Autodesk Inventor part; units mm, degrees
ref_plane "Work Plane1" through (29, 0, 0) normal (0, -1, 0) x (1, 0, 0)
ref_plane "YZ Plane" through (0, 0, 0) normal (1, 0, 0) x (0, 1, 0)
ref_plane "XZ Plane" through (0, 0, 0) normal (0, 1, 0) x (-1, 0, 0)
sketch "Sketch1" plane through (0, 0, 0) normal (0, 0, 1) x (1, 0, 0)
  line L0 (-0.19, 0) -> (20, 0)
  line L1 (20, 0) -> (20, 2.5)
  line L2 (20, 2.5) -> (2.4, 2.5)
  line L3 (2.4, 2.5) -> (1.9091, 2.5)
  line L4 (1.9091, 2.5) -> (0, 2.5)
  line L5 (0, 2.5) -> (0, 4.75)
  line L6 (0, 4.75) -> (-2.75, 4.75)
  line L7 (-2.75, 4.75) -> (-2.75, 1.7321)
  line L8 (-2.75, 1.7321) -> (-1.19, 1.7321)
  line L9 (-1.19, 1.7321) -> (-0.19, 0)
  line L10 (-7.3, 0) -> (24.55, 0)
  line L11 (0, -0.95) -> (0, 5.7)
  line L12 (2.4, 2.5) -> (0, 2.5) construction
  dimension "d1" = 17.6
  dimension "d2" = 0.4909
  dimension "d3" = 2.75
  dimension "d4" = 1.56
  dimension "d5" = 60
  dimension "d6" = 5
  dimension "d7" = 5
  dimension "d8" = 3.4641
  dimension "d9" = 9.5
  dimension "d26" = 20
revolve "Body" add sketch "Sketch1" angle 360 about axis through (-0.19, 0, 0) along (1, 0, 0)
sketch "Sketch2" plane through (-2.75, 0, 0) normal (-1, 0, 0) x (0, 0, 1)
  circle A0 centre (0, 0) radius 1.7321
  line L0 (0, -6.65) -> (0, 6.65)
  line L1 (-6.65, 0) -> (6.65, 0)
  line L2 (1.7321, 0) -> (0.866, -1.5)
  line L3 (0.866, -1.5) -> (-0.866, -1.5)
  line L4 (-0.866, -1.5) -> (-1.7321, 0)
  line L5 (-1.7321, 0) -> (-0.866, 1.5)
  line L6 (-0.866, 1.5) -> (0.866, 1.5)
  line L7 (0.866, 1.5) -> (1.7321, 0)
extrude "Slot" add sketch "Sketch2" against normal up to next contours L7 A0 | A0 L2 | L6 L0 A0 | A0 L0 L3 | L0 L6 A0 | A0 L3 L0 | L4 A0 | A0 L5
fillet "Fillet1" radius 2.37 1 edges at (-2.75, -4.75, 0)
thread "Thread"
chamfer "Chamfer1" distance 0.4908 distance2 0.4908 1 edges at (20, -2.5, 0) measured on face at (20, -0.7379, -0.3873)
ref_plane "Work Plane1" through (29, 0, 0) normal (0, -1, 0) x (1, 0, 0)
fillet "Fillet2" radius 0.45 1 edges at (0, -2.5, 0)
equation "\"d1\" = GEL"
equation "\"d3\" = KOH"
equation "\"d4\" = INTI"
equation "\"d6\" = GD"
equation "\"d7\" = BDM"
equation "\"d8\" = 1.1547 * SW"
equation "\"d9\" = KOD"
equation "\"d26\" = NLG"
equation "\"d30\" = R"
equation "\"d17\" = RR"
equation "\"d13\" = GEL"
equation "\"d15\" = -0.5 * SPD + 0.5 * GD"
equation "\"d16\" = GUL"
equation "\"GD\" = NND"
equation "\"NLG\" = 20"
equation "\"GEL\" = 17.6"
equation "\"KOD\" = 9.5"
equation "\"KOH\" = 2.75"
equation "\"INTI\" = 1.56"
equation "\"GAL\" = 0.61345 * PTC"
equation "\"GUL\" = 0.61345 * PTC"
equation "\"BDM\" = NND"
equation "\"SW\" = 3"
equation "\"RR\" = 2.37"
equation "\"SPD\" = NND - 1.2269 * PTC"
equation "\"R\" = 0.45"
equation "\"TOA\" = 30deg"
equation "\"GD1\" = THREADDIA - 1.2269 * PTC"
equation "\"THREADDIA\" = 5"
equation "\"PTC\" = 0.8"
equation "\"NND\" = 5"
equation "\"KOH1\" = 0.38"
equation "\"E0\" = 3.443"
properties part number "ISO 7380-1 - M5 x 20" material "Steel"
The model under review builds one solid part; all positions refer to its coordinate system, in mm. A direction names the side the tool comes from. Round coordinates to 2 decimals unless told otherwise and drop trailing zeros. Loops run counter-clockwise (first coordinate to the right, second up) from the corner with the lowest first, then second, coordinate; pieces in that order, holes last.
1) Wall thickness on line 1 along Y through (x, z) = (13.5, -0.75); line 2 along Z through (x, y) = (6.5, 0.5); line 3 along X through (y, z) = (2.5, 2.5): over which ranges is each line inside the solid? List them lowest first.
Values follow:
line 1: y = -2.38 to 2.38
line 2: z = -2.45 to 2.45
line 3: x = -2.45 to 0
2) Clearance check with flat-ended pins moving along their axes: P1, Ø5, axis at y = 1.5, z = 2.5, coming from the -X side; P2, Ø1.4, axis at x = -2, z = 0.5, coming from the -Y side; P3, Ø1.4, axis at x = -1.5, z = 0.5, coming from the +Y side. State where each tip first meets the part, or that it passes through.
Values follow:
P1: stops at x = -2.75
P2: stops at y = -4.54
P3: stops at y = 4.7
3) The part is to be moulded in two halves that separate along Z. For faces 4 (the face through (20, 0, 0)), 5 (the face through (-1.915, 0.761, 1.293)), 6 (the face through (-2, 1.5, 0)), 7 (the face through (9.85, -0.54, 2.44)), say which applies: pulls with the +Z half, pulls with the -Z half, needs draft (parallel to the pull), parting line crosses it, or undercut.
Values follow:
face 4: needs draft
face 5: undercut
face 6: undercut
face 7: parting line crosses it
4) Consider section A-A on x = 2.75. State the section outline as (y, z) points.
Values follow:
outline: circle Ø5 at (0, 0)
5) Tool access review of faces 1 (the face through (-2, -1.5, 0)), 2 (the face through (-0.193, 2.192, 4.214)), 3 (the face through (0, -0.1, -3.1)): name each direction out of +Z, -Z, +X, -X, +Y, -Y from which nothing blocks a thin tool from reaching the whole face with its end or side.
Values follow:
face 1: -X
face 2: +X, -X
face 3: +X
